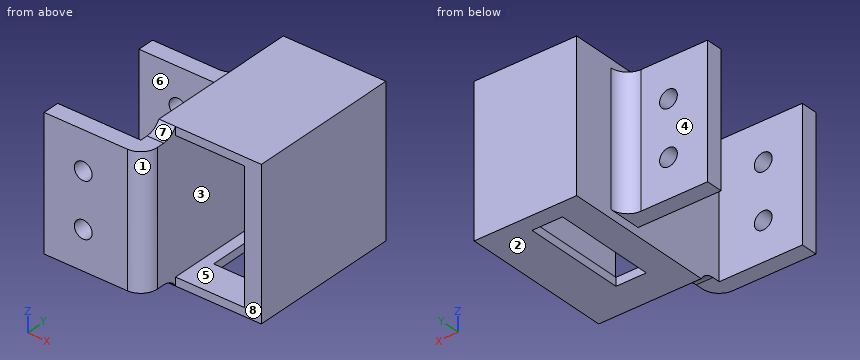
from build123d import *

# Parameters (mm, degrees)
SKETCH1_W                = 26.6
SKETCH1_H                = 27.6
SKETCH1_W_2              = 23.6
SKETCH1_H_2              = 24.6
BOSS_EXTRUDE1_DEPTH      = 12.5
SKETCH2_W                = 26.6
SKETCH2_H                = 27.6
BOSS_EXTRUDE2_DEPTH      = 3
SKETCH4_W                = 26.6
SKETCH4_H                = 27.6
BOSS_EXTRUDE3_DEPTH      = 3
SKETCH6_W                = 12.5
SKETCH6_H                = 20.6
CUT_EXTRUDE1_DEPTH       = 3
BOSS_EXTRUDE4_DEPTH      = 7
BOSS_EXTRUDE4_DEPTH_BACK = 17
SKETCH7_W                = 12.54
SKETCH7_H                = 14.392021094
SKETCH8_R                = 1.6
CUT_EXTRUDE2_DEPTH       = 41.17835238
SKETCH10_W               = 9.54
SKETCH10_H               = 18
CUT_EXTRUDE3_DEPTH       = 34.198989028
SKETCH14_W               = 12.5
SKETCH14_H               = 23.6
CUT_EXTRUDE5_DEPTH       = 3
SKETCH24_W               = 3
SKETCH24_H               = 5.880857343
BOSS_EXTRUDE7_DEPTH      = 7
SKETCH25_W               = 3
SKETCH25_H               = 6.327121563
BOSS_EXTRUDE8_DEPTH      = 7
SKETCH27_W               = 26.6
SKETCH27_H               = 3
BOSS_EXTRUDE9_DEPTH      = 20
SKETCH32_W               = 26.6
SKETCH32_H               = 3
BOSS_EXTRUDE10_DEPTH     = 20
FILLET1_R                = 3
SKETCH35_W               = 20
SKETCH35_H               = 24
CUT_EXTRUDE9_DEPTH       = 1.5
SKETCH36_W               = 3
SKETCH36_H               = 7
CUT_EXTRUDE10_DEPTH      = 1.5
SKETCH37_W               = 20
SKETCH37_H               = 24
CUT_EXTRUDE11_DEPTH      = 1.5
SKETCH38_W               = 3
SKETCH38_H               = 7
CUT_EXTRUDE12_DEPTH      = 1.5
FILLET3_R                = 3
FILLET4_R                = 3
FILLET5_R                = 3
SKETCH39_W               = 5
SKETCH39_H               = 23.6
CUT_EXTRUDE13_DEPTH      = 24
SKETCH41_R               = 1.6
CUT_EXTRUDE14_DEPTH      = 24
SKETCH42_W               = 5.5
SKETCH42_H               = 18.6
CUT_EXTRUDE15_DEPTH      = 38.237749663


with BuildPart() as part:
    # Sketch1 → Boss-Extrude1 (new body)
    with BuildSketch(Plane(origin=(0, 0, 0), x_dir=(0, 0, -1), z_dir=(1, 0, 0))):
        Rectangle(SKETCH1_W, SKETCH1_H)
        Rectangle(SKETCH1_W_2, SKETCH1_H_2, mode=Mode.SUBTRACT)
    extrude(amount=BOSS_EXTRUDE1_DEPTH)

    # Sketch2 → Boss-Extrude2 (add)
    with BuildSketch(Plane.ZY):
        Rectangle(SKETCH2_W, SKETCH2_H)
    extrude(amount=BOSS_EXTRUDE2_DEPTH)

    # Sketch4 → Boss-Extrude3 (add)
    with BuildSketch(Plane(origin=(12.5, 0, 0), x_dir=(0, 0, -1), z_dir=(1, 0, 0))):
        Rectangle(SKETCH4_W, SKETCH4_H)
    extrude(amount=BOSS_EXTRUDE3_DEPTH)

    # Sketch6 → Cut-Extrude1 (cut)
    with BuildSketch(Plane(origin=(0, -13.8, 0), x_dir=(-1, 0, 0), z_dir=(0, -1, 0))):
        with Locations((-6.25, 0)):
            Rectangle(SKETCH6_W, SKETCH6_H)
    extrude(amount=-CUT_EXTRUDE1_DEPTH, mode=Mode.SUBTRACT)

    # Sketch7 → Boss-Extrude4 (add, two sides: drawn at the far end of the back side and taken through both)
    with BuildSketch(Plane(origin=(0, -13.8, 0), x_dir=(-1, 0, 0), z_dir=(0, -1, 0)).offset(-BOSS_EXTRUDE4_DEPTH_BACK)):
        with Locations((6.27, -0.22313211)):
            Rectangle(SKETCH7_W, SKETCH7_H)
    extrude(amount=BOSS_EXTRUDE4_DEPTH + BOSS_EXTRUDE4_DEPTH_BACK)

    # Sketch8 → Cut-Extrude2 (cut, through all)
    with BuildSketch(Plane(origin=(0, -20.8, 0), x_dir=(-1, 0, 0), z_dir=(0, -1, 0))):
        with Locations(Location((9.94, -4.900507757, 0), (0, 0, 90))):
            Circle(SKETCH8_R)
        with Locations(Location((9.94, 4.836704631, 0), (0, 0, 90))):
            Circle(SKETCH8_R)
    extrude(amount=-CUT_EXTRUDE2_DEPTH, mode=Mode.SUBTRACT)

    # Sketch10 → Cut-Extrude3 (cut, through all)
    with BuildSketch(Plane.XY.offset(7.419142657)):
        with Locations((-7.77, -8.8)):
            Rectangle(SKETCH10_W, SKETCH10_H)
    extrude(amount=-CUT_EXTRUDE3_DEPTH, mode=Mode.SUBTRACT)

    # Sketch14 → Cut-Extrude5 (cut)
    with BuildSketch(Plane(origin=(0, -13.8, 0), x_dir=(-1, 0, 0), z_dir=(0, -1, 0))):
        with Locations((-6.25, 0)):
            Rectangle(SKETCH14_W, SKETCH14_H)
    extrude(amount=-CUT_EXTRUDE5_DEPTH, mode=Mode.SUBTRACT)

    # Sketch24 → Boss-Extrude7 (add)
    with BuildSketch(Plane(origin=(0, -13.8, 0), x_dir=(-1, 0, 0), z_dir=(0, -1, 0))):
        with Locations((1.5, -10.359571328)):
            Rectangle(SKETCH24_W, SKETCH24_H)
    extrude(amount=BOSS_EXTRUDE7_DEPTH)

    # Sketch25 → Boss-Extrude8 (add)
    with BuildSketch(Plane(origin=(0, -13.8, 0), x_dir=(-1, 0, 0), z_dir=(0, -1, 0))):
        with Locations((1.5, 10.136439219)):
            Rectangle(SKETCH25_W, SKETCH25_H)
    extrude(amount=BOSS_EXTRUDE8_DEPTH)

    # Sketch27 → Boss-Extrude9 (add)
    with BuildSketch(Plane.ZY.offset(3)):
        with Locations((0, -19.3)):
            Rectangle(SKETCH27_W, SKETCH27_H)
    extrude(amount=BOSS_EXTRUDE9_DEPTH)

    # Sketch32 → Boss-Extrude10 (add)
    with BuildSketch(Plane.ZY.offset(3)):
        with Locations((0, 1.7)):
            Rectangle(SKETCH32_W, SKETCH32_H)
    extrude(amount=BOSS_EXTRUDE10_DEPTH)

    # Fillet1
    fillet1_edges = [part.edges().sort_by_distance(p)[0] for p in [
        (0, -20.8, 0),
    ]]
    fillet(fillet1_edges, radius=FILLET1_R)

    # Sketch35 → Cut-Extrude9 (cut)
    with BuildSketch(Plane.XY.offset(13.3)):
        with Locations((-13, -8.8)):
            Rectangle(SKETCH35_W, SKETCH35_H)
    extrude(amount=-CUT_EXTRUDE9_DEPTH, mode=Mode.SUBTRACT)

    # Sketch36 → Cut-Extrude10 (cut)
    with BuildSketch(Plane.XY.offset(13.3)):
        with Locations((-1.5, -17.3)):
            Rectangle(SKETCH36_W, SKETCH36_H)
    extrude(amount=-CUT_EXTRUDE10_DEPTH, mode=Mode.SUBTRACT)

    # Sketch37 → Cut-Extrude11 (cut)
    with BuildSketch(Plane(origin=(0, 0, -13.3), x_dir=(-1, 0, 0), z_dir=(0, 0, -1))):
        with Locations((13, -8.8)):
            Rectangle(SKETCH37_W, SKETCH37_H)
    extrude(amount=-CUT_EXTRUDE11_DEPTH, mode=Mode.SUBTRACT)

    # Sketch38 → Cut-Extrude12 (cut)
    with BuildSketch(Plane(origin=(0, 0, -13.3), x_dir=(-1, 0, 0), z_dir=(0, 0, -1))):
        with Locations((1.5, -17.3)):
            Rectangle(SKETCH38_W, SKETCH38_H)
    extrude(amount=-CUT_EXTRUDE12_DEPTH, mode=Mode.SUBTRACT)

    # Fillet3
    # the kernel refuses this fillet: 3 mm, written as the material it adds along each edge
    with BuildSketch(Plane(origin=(-3, -13.8, 11.8), x_dir=(0, 0, 1), z_dir=(1, 0, 0))) as fillet3_piece_1:
        with BuildLine():
            CenterArc((3, 2.598076211), FILLET3_R, 180, 60)
            Line((0, 2.598076211), (0, 0))
            Line((0, 0), (1.5, 0))
        make_face()
    extrude(amount=3)

    # Fillet4
    # the kernel refuses this fillet: 3 mm, written as the material it adds along each edge
    with BuildSketch(Plane(origin=(0, -13.8, -11.8), x_dir=(0, 0, -1), z_dir=(-1, 0, 0))) as fillet4_piece_1:
        with BuildLine():
            CenterArc((3, 2.598076211), FILLET4_R, 180, 60)
            Line((0, 2.598076211), (0, 0))
            Line((0, 0), (1.5, 0))
        make_face()
    extrude(amount=3)

    # Fillet5
    fillet5_edges = [part.edges().sort_by_distance(p)[0] for p in [
        (-3, 3.2, 0),
    ]]
    fillet(fillet5_edges, radius=FILLET5_R)

    # Sketch39 → Cut-Extrude13 (cut)
    with BuildSketch(Plane(origin=(0, -20.8, 0), x_dir=(-1, 0, 0), z_dir=(0, -1, 0))):
        with Locations((20.5, 0)):
            Rectangle(SKETCH39_W, SKETCH39_H)
    extrude(amount=-CUT_EXTRUDE13_DEPTH, mode=Mode.SUBTRACT)

    # Sketch41 → Cut-Extrude14 (cut)
    with BuildSketch(Plane(origin=(0, -20.8, 0), x_dir=(-1, 0, 0), z_dir=(0, -1, 0))):
        with Locations(Location((10.94, -4.900507757, 0), (0, 0, 90))):
            Circle(SKETCH41_R)
        with Locations(Location((10.94, 4.836704631, 0), (0, 0, 90))):
            Circle(SKETCH41_R)
    extrude(amount=-CUT_EXTRUDE14_DEPTH, mode=Mode.SUBTRACT)

    # Sketch42 → Cut-Extrude15 (cut, through all)
    with BuildSketch(Plane(origin=(0, 0, 11.8), x_dir=(-1, 0, 0), z_dir=(0, 0, -1))):
        with Locations((-4.75, 1.5)):
            Rectangle(SKETCH42_W, SKETCH42_H)
    extrude(amount=CUT_EXTRUDE15_DEPTH, mode=Mode.SUBTRACT)


solid = part.part
Work out the finished part from the listing and answer in its coordinate system (mm). Face numbers are marked on the shaded views. A direction names the side the tool comes from. Give positions to 0.01 mm unless a question says otherwise; leave off trailing zeros. Write each loop counter-clockwise with the first axis right and the second up, starting at its lowest first coordinate (ties: lowest second). Pieces come first, ordered by that corner, then holes. Notation, with made-up numbers: (80.25, 54.25) - (131.25, 54.25) arc R12 cw to (131.25, 65.25) - close; hole circle Ø5 at (-2.5, 82). An arc over 180 degrees is marked (long way). One line per item, written item: value. Start each with the question number.
1. For the marked faces 4, 5, 6, 7 and 8, determine the directions among +Z, -Z, +X, -X, +Y, -Y from which every point of the face is accessible in a straight line to the end or side of a thin tool.
2. For a pull along Z with two mould halves and no side action, classify the marked faces 1, 2 and 3 as +Z half, -Z half, draft (parallel to the pull), parting line (faces both ways), or undercut.
3. Given pin 1 (1 mm diameter, centred on x = 4.5, z = -2.5, fed in from -Y); pin 2 (1.3 mm diameter, centred on x = -11.5, y = -18, fed in from +Z); pin 3 (2 mm diameter, centred on x = -11, y = 3, fed in from -Z), each flat-ended and moving along its own axis, determine where each tip first touches the part or whether it passes through.
4. Find section C-C (z = -5.25). Write down the section's boundary in (x, y), then the cut area to 3 significant figures.
5. Find section B-B (x = -10.94). Write down the section's boundary in (y, z), then the cut area to 3 significant figures.
6. Consider probe 1 along Z at (x, y) = (11, -9.5); probe 2 along Y at (x, z) = (-8.5, 7.75); probe 3 along X at (y, z) = (1.5, 1.25). Determine where each line is inside the solid, lowest interval first.
7. Find section D-D (x = 9). Write down the section's boundary in (y, z), then the cut area to 3 significant figures.
8. Find section A-A (y = -12). Write down the section's boundary in (x, z), then the cut area to 3 significant figures.
Geometry results:
1. face 4: +Z, -Z, -X, +Y
1. face 5: -Y
1. face 6: +Z, -Z, -X
1. face 7: +Z, +X, -X, -Y
1. face 8: +Z, -Z, +X, -Y
2. face 1: draft
2. face 2: -Z half
2. face 3: undercut
3. pin 1: y = 12.3
3. pin 2: z = 11.8
3. pin 3: z = -11.8
4. outline: (-18, -20.8) - (-12.49, -20.8) - (-12.49, -17.8) - (-18, -17.8) - close; (-18, 0.2) - (-12.49, 0.2) - (-12.49, 3.2) - (-18, 3.2) - close; (-9.39, -20.8) - (-3, -20.8) arc R3 ccw to (0, -17.8) - (0, 12.3) - (12.5, 12.3) - (12.5, -13.8) - (15.5, -13.8) - (15.5, 13.8) - (-3, 13.8) - (-3, 6.2) arc R3 cw to (-6, 3.2) - (-9.39, 3.2) - (-9.39, 0.2) - (-3, 0.2) - (-3, -17.8) - (-9.39, -17.8) - close
4. area: 277 mm2
5. outline: (-20.8, -11.8) - (-17.8, -11.8) - (-17.8, -6.44) - (-20.8, -6.44) - close; (-20.8, -3.24) - (-17.8, -3.24) - (-17.8, 3.3) - (-20.8, 3.3) - close; (-20.8, 6.5) - (-17.8, 6.5) - (-17.8, 11.8) - (-20.8, 11.8) - close; (0.2, -11.8) - (3.2, -11.8) - (3.2, -6.44) - (0.2, -6.44) - close; (0.2, -3.24) - (3.2, -3.24) - (3.2, 3.3) - (0.2, 3.3) - close; (0.2, 6.5) - (3.2, 6.5) - (3.2, 11.8) - (0.2, 11.8) - close
5. area: 103 mm2
6. probe 1: -13.3 to -11.8, 11.8 to 13.3
6. probe 2: -20.8 to -17.8, 0.2 to 3.2
6. probe 3: -18 to 0, 12.5 to 15.5
7. outline: (-13.8, -13.3) - (13.8, -13.3) - (13.8, 13.3) - (-13.8, 13.3) - (-13.8, 11.8) - (12.3, 11.8) - (12.3, -11.8) - (-13.8, -11.8) - close
7. area: 118 mm2
8. outline: (-3, -13.3) - (15.5, -13.3) - (15.5, 13.3) - (-3, 13.3) - close; hole (0, -11.8) - (12.5, -11.8) - (12.5, 11.8) - (0, 11.8) - close
8. area: 197 mm2
